```python
from build123d import *

# Parameters (mm, degrees)
BOSS_EXTRUDE1_DEPTH                            = 2.9
SKETCH2_W                                      = 2.75
SKETCH2_H                                      = 83.9
BOSS_EXTRUDE2_DEPTH                            = 20.9
CUT_EXTRUDE1_DEPTH                             = 27.75
CSK_FOR_M6_FLAT_HEAD_MACHINE_SCREW1_AT_2_COUNT = 2
CSK_FOR_M6_FLAT_HEAD_MACHINE_SCREW1_AT_2_PITCH = 59.791303716
SKETCH8_W                                      = 41.834673512
SKETCH8_H                                      = 83.9
CUT_REVOLVE4_ANGLE                             = 3


with BuildPart() as part:
    # Sketch1 → Boss-Extrude1 (new body)
    with BuildSketch(Plane.XY):
        with BuildLine():
            Line((-15.4, -41.95), (20.4, -41.95))
            Line((20.4, -41.95), (20.4, 41.95))
            Line((20.4, 41.95), (-15.4, 41.95))
            ThreePointArc((-15.4, 41.95), (-18.935533906, 40.485533906), (-20.4, 36.95))
            Line((-20.4, 36.95), (-20.4, -36.95))
            ThreePointArc((-20.4, -36.95), (-18.935533906, -40.485533906), (-15.4, -41.95))
        make_face()
    extrude(amount=BOSS_EXTRUDE1_DEPTH)

    # Sketch2 → Boss-Extrude2 (add)
    with BuildSketch(Plane.XY.offset(2.9)):
        with Locations((19.025, 0)):
            Rectangle(SKETCH2_W, SKETCH2_H)
    extrude(amount=BOSS_EXTRUDE2_DEPTH)

    # Sketch4 → Cut-Extrude1 (cut)
    with BuildSketch(Plane(origin=(20.4, 0, 0), x_dir=(0, 0, -1), z_dir=(1, 0, 0))):
        with BuildLine():
            Line((-23.8, 36.676506119), (-23.8, 41.95))
            Line((-23.8, 41.95), (-18.526506119, 41.95))
            ThreePointArc((-18.526506119, 41.95), (-22.255429403, 40.405429403), (-23.8, 36.676506119))
        make_face()
        with BuildLine():
            Line((-23.8, -41.95), (-23.8, -36.676506119))
            ThreePointArc((-23.8, -36.676506119), (-22.255429403, -40.405429403), (-18.526506119, -41.95))
            Line((-18.526506119, -41.95), (-23.8, -41.95))
        make_face()
    extrude(amount=-CUT_EXTRUDE1_DEPTH, mode=Mode.SUBTRACT)

    # Sketch6 → CSK for M6 Flat Head Machine Screw1 (revolve, cut)
    with BuildSketch(Plane(origin=(2.5, 29.895651858, 0), x_dir=(0, 1, 0), z_dir=(1, 0, 0))):
        Polygon((0, 0), (0, 2.9), (3.3, 2.9), (3.3, 3), (6.3, 0), align=None)
    csk_for_m6_flat_head_machine_screw1 = revolve(axis=Axis((2.5, 29.895651858, -6.35), (0, 0, 1)), mode=Mode.SUBTRACT)

    # CSK for M6 Flat Head Machine Screw1 at 2: CSK for M6 Flat Head Machine Screw1 ×2
    with Locations(*[(0, -i * CSK_FOR_M6_FLAT_HEAD_MACHINE_SCREW1_AT_2_PITCH, 0) for i in range(1, CSK_FOR_M6_FLAT_HEAD_MACHINE_SCREW1_AT_2_COUNT)]):
        add(csk_for_m6_flat_head_machine_screw1, mode=Mode.SUBTRACT)

    # Sketch8 → Cut-Revolve4 (revolve, cut)
    with BuildSketch(Plane(origin=(20.4, 0, 0), x_dir=(0, 0, -1), z_dir=(1, 0, 0))):
        with Locations((-20.917336756, 0)):
            Rectangle(SKETCH8_W, SKETCH8_H)
    revolve(axis=Axis((20.4, -41.95, 0), (0, -1, 0)), revolution_arc=CUT_REVOLVE4_ANGLE, mode=Mode.SUBTRACT)


solid = part.part
```
Model file for the job. Use its own axes, mm. A direction names the side the tool comes from. Coordinates: 2 decimals unless noted, no trailing zeros. Order: outer loops, then holes, each group sorted by start corner. A loop starts at its lowest first (then second) coordinate and runs counter-clockwise, first axis right, second up. Notation, with made-up numbers: (45.25, 59) - (49.25, 59) arc R23 cw to (49.25, 71) - close; hole circle Ø10 at (33.5, 28.5). An arc over 180 degrees is marked (long way). Return JSON: item names as keys, results as strings. Group by question number.
1) Saw through at C-C, the plane x = -12. Write the cut outline in (y, z).
2) Saw through at B-B, the plane y = 17. Write the cut outline in (x, z), plus the area to 3 significant figures.
3) Saw through at A-A, the plane x = 2.5. Write the cut outline in (y, z).
4) Flat gauge pins, fed straight in: P1, Ø19, axis at x = -10, y = 19.5, coming from the +Z side; P2, Ø6.5, axis at y = -7, z = 15, coming from the -X side; P3, Ø6, axis at y = -3, z = 20.5, coming from the +X side. Where does each tip first touch, or does it go through?
5) Mould opens along X. For faces 1 (the flat face through (19.768, 0.587, 12.067)), 2 (the flat face through (0, 1, 0)), 3 (the conical face through (4.679, -32.738, 2.719)), 4 (the flat face through (-20.4, 1, 1)) say: released by +X, released by -X, zero draft, split by the parting line, or undercut.
6) Probe line 1 (Z direction, x = -8.5, y = -11); line 2 (X direction, y = 24, z = 13); line 3 (X direction, y = -32, z = 7.5). List the from-to ranges inside material, lowest first. Write a range as from..to.
7) Saw through at D-D, the plane z = 21. Write the cut outline in (x, y), plus the area to 3 significant figures.
8) Tool access for faces 5 (the cylindrical face through (-18.9, 40.52, 1.43)), 6 (the flat face through (17.65, -1, 13)): list every direction of +Z, -Z, +X, -X, +Y, -Y with a clear straight run to the whole face (end or side of a thin tool).
Values found:
{
 "1": {"outline": "(-41.95, 0) - (41.95, 0) - (41.95, 2.9) - (-41.95, 2.9) - close"},
 "2": {"outline": "(-20.4, 0) - (20.4, 0) - (19.15, 23.8) - (17.65, 23.8) - (17.65, 2.9) - (-20.4, 2.9) - close", "area": "161 mm²"},
 "3": {"outline": "(-41.95, 0) - (-36.2, 0) - (-33.3, 2.9) - (-41.95, 2.9) - close; (-26.5, 2.9) - (-23.6, 0) - (23.6, 0) - (26.5, 2.9) - close; (33.3, 2.9) - (36.2, 0) - (41.95, 0) - (41.95, 2.9) - close"},
 "4": {"P1": "stops at z = 2.9", "P2": "stops at x = 17.65", "P3": "stops at x = 19.48"},
 "5": {"face 1": "released by +X", "face 2": "zero draft", "face 3": "undercut", "face 4": "released by -X"},
 "6": {"line 1": "z = 0..2.9", "line 2": "x = 17.65..19.72", "line 3": "x = 17.65..20.01"},
 "7": {"outline": "(17.65, -41.33) - (19.3, -41.33) - (19.3, 41.33) - (17.65, 41.33) - close", "area": "136 mm²"},
 "8": {"face 5": "+Z, -Z, -X, +Y", "face 6": "+Z, -X, +Y, -Y"}
}
